Design review of the part built by this model. Coordinates are the model's own, in mm. A direction names the side the tool comes from. Coordinates: 2 decimals unless noted, no trailing zeros. Order: outer loops, then holes, each group sorted by start corner. A loop starts at its lowest first (then second) coordinate and runs counter-clockwise, first axis right, second up. Notation, with made-up numbers: M 59,45.5 L 93,45.5 A18 ccw 93,69.5 Z; hole C 81.5,-30.75 d11. An arc over 180 degrees is marked long. Answer as a JSON object with one key per item and string values.
from build123d import *

# Parameters (mm, degrees)
SKETCH1_W               = 40.3
SKETCH1_H               = 19.5
BOSS_EXTRUDE1_DEPTH     = 27
SKETCH2_W               = 54
SKETCH2_H               = 19.5
BOSS_EXTRUDE2_DEPTH     = 2.5
SKETCH3_W               = 40.3
SKETCH3_H               = 19.5
BOSS_EXTRUDE3_DEPTH     = 6.5
SKETCH4_R               = 2.75
BOSS_EXTRUDE4_DEPTH     = 8
CUT_EXTRUDE1_DEPTH      = 42.162027404
CUT_EXTRUDE1_DEPTH_BACK = 42.162027404
SKETCH5_R               = 2
BOSS_EXTRUDE5_DEPTH     = 3
SKETCH7_R               = 6.5
BOSS_EXTRUDE6_DEPTH     = 2
BOSS_EXTRUDE7_DEPTH     = 3


with BuildPart() as part:
    # Sketch1 → Boss-Extrude1 (new body)
    with BuildSketch(Plane(origin=(0, 0, 0), x_dir=(1, 0, 0), z_dir=(0, 1, 0))):
        Rectangle(SKETCH1_W, SKETCH1_H)
    extrude(amount=BOSS_EXTRUDE1_DEPTH)

    # Sketch2 → Boss-Extrude2 (add)
    with BuildSketch(Plane(origin=(0, 27, 0), x_dir=(1, 0, 0), z_dir=(0, 1, 0))):
        Rectangle(SKETCH2_W, SKETCH2_H)
    extrude(amount=BOSS_EXTRUDE2_DEPTH)

    # Sketch3 → Boss-Extrude3 (add)
    with BuildSketch(Plane(origin=(0, 29.5, 0), x_dir=(1, 0, 0), z_dir=(0, 1, 0))):
        Rectangle(SKETCH3_W, SKETCH3_H)
    extrude(amount=BOSS_EXTRUDE3_DEPTH)

    # Sketch4 → Boss-Extrude4 (add)
    with BuildSketch(Plane(origin=(0, 36, 0), x_dir=(1, 0, 0), z_dir=(0, 1, 0))):
        with Locations(Location((9.85, 0, 0), (0, 0, 270))):
            Circle(SKETCH4_R)
    extrude(amount=BOSS_EXTRUDE4_DEPTH)

    # Sketch5 → Cut-Extrude1 (cut, two sides: drawn at the far end of the back side and taken through both)
    with BuildSketch(Plane(origin=(0, 29.5, 0), x_dir=(1, 0, 0), z_dir=(0, 1, 0)).offset(-CUT_EXTRUDE1_DEPTH_BACK)):
        with Locations(Location((-24.315, 5, 0), (0, 0, 270))):
            Circle(SKETCH5_R)
        with Locations(Location((-24.315, -5, 0), (0, 0, 270))):
            Circle(SKETCH5_R)
        with Locations(Location((24.315, -5, 0), (0, 0, 270))):
            Circle(SKETCH5_R)
        with Locations(Location((24.315, 5, 0), (0, 0, 270))):
            Circle(SKETCH5_R)
    extrude(amount=CUT_EXTRUDE1_DEPTH + CUT_EXTRUDE1_DEPTH_BACK, mode=Mode.SUBTRACT)

    # Sketch6 → Boss-Extrude5 (add)
    with BuildSketch(Plane(origin=(0, 36, 0), x_dir=(1, 0, 0), z_dir=(0, 1, 0))):
        with BuildLine():
            Line((9.85, -9.75), (-13.85, -9.75))
            Line((-13.85, -9.75), (-13.85, 9.75))
            Line((-13.85, 9.75), (9.85, 9.75))
            ThreePointArc((9.85, 9.75), (19.6, 0), (9.85, -9.75))
        make_face()
    extrude(amount=BOSS_EXTRUDE5_DEPTH)

    # Sketch7 → Boss-Extrude6 (add)
    with BuildSketch(Plane(origin=(0, 39, 0), x_dir=(1, 0, 0), z_dir=(0, 1, 0))):
        with Locations(Location((9.85, 0, 0), (0, 0, 270))):
            Circle(SKETCH7_R)
    extrude(amount=BOSS_EXTRUDE6_DEPTH)

    # Sketch8 → Boss-Extrude7 (add)
    with BuildSketch(Plane(origin=(0, 36, 0), x_dir=(1, 0, 0), z_dir=(0, 1, 0))):
        with BuildLine():
            Line((-13.85, 4.510933332), (-13.85, -4.510933332))
            ThreePointArc((-13.85, -4.510933332), (-15.530301972, 0), (-13.85, 4.510933332))
        make_face()
    extrude(amount=BOSS_EXTRUDE7_DEPTH)


solid = part.part
1) Tool access review of faces 4 (the flat face through (24, 29.5, 0)), 5 (the cylindrical face through (19.598, 37.479, -0.214)), 6 (the cylindrical face through (-15.53, 37.48, 0.07)): name each direction out of +Z, -Z, +X, -X, +Y, -Y from which nothing blocks a thin tool from reaching the whole face with its end or side.
Taken from the geometry:
{"face 4": "+Z, -Z, +X, +Y", "face 5": "+X, +Y", "face 6": "-X, +Y"}
2) Add section C-C (x = 6). State the section outline as (y, z) points, and give its area (3 significant figures).
Taken from the geometry:
{"outline": "M 0,-9.75 L 39,-9.75 L 39,-5.24 L 41,-5.24 L 41,5.24 L 39,5.24 L 39,9.75 L 0,9.75 Z", "area": "781 mm2"}
3) Mouldability with a two-part tool opening along Z and no side actions: class faces 1 (the cylindrical face through (-22.33, 28.23, -5.26)), 2 (the flat face through (20.15, 13, 0)), 3 (the flat face through (0, 19, -9.75)) as released by +Z, released by -Z, zero draft, split by the parting line, or undercut.
Taken from the geometry:
{"face 1": "undercut", "face 2": "zero draft", "face 3": "released by -Z"}
4) Add section A-A (z = 0). State the section outline as (x, y) points.
Taken from the geometry:
{"outline": "M -27,27 L -20.15,27 L -20.15,0 L 20.15,0 L 20.15,27 L 27,27 L 27,29.5 L 20.15,29.5 L 20.15,36 L 19.6,36 L 19.6,39 L 16.35,39 L 16.35,41 L 12.6,41 L 12.6,44 L 7.1,44 L 7.1,41 L 3.35,41 L 3.35,39 L -15.53,39 L -15.53,36 L -20.15,36 L -20.15,29.5 L -27,29.5 Z"}
5) Insertion check: pin 1 Ø8 at (x, z) = (-5, -3.5) entering from -Y; pin 2 Ø2 at (x, z) = (-23, -0.5) entering from -Y; pin 3 Ø10 at (x, z) = (-21, 6.5) entering from +Y; pin 4 Ø6 at (y, z) = (7, 5) entering from +X. Each pin has a flat end and moves straight along its axis. Give the tip position at first contact, or say it passes through.
Taken from the geometry:
{"pin 1": "stops at y = 0", "pin 2": "stops at y = 27", "pin 3": "stops at y = 36", "pin 4": "stops at x = 20.15"}
6) Add section B-B (z = 5.25). State the section outline as (x, y) points, and give its area (3 significant figures).
Taken from the geometry:
{"outline": "M -27,27 L -26.3,27 L -26.3,29.5 L -27,29.5 Z; M -22.33,27 L -20.15,27 L -20.15,0 L 20.15,0 L 20.15,27 L 22.33,27 L 22.33,29.5 L 20.15,29.5 L 20.15,36 L 18.07,36 L 18.07,39 L 13.68,39 L 13.68,41 L 6.02,41 L 6.02,39 L -13.85,39 L -13.85,36 L -20.15,36 L -20.15,29.5 L -22.33,29.5 Z; M 26.3,27 L 27,27 L 27,29.5 L 26.3,29.5 Z", "area": "1,580 mm2"}
7) Add section D-D (y = 25). State the section outline as (x, z) points.
Taken from the geometry:
{"outline": "M -20.15,-9.75 L 20.15,-9.75 L 20.15,9.75 L -20.15,9.75 Z"}
8) To check wall thickness, follow L1, parallel to X at y = 28.05, z = 5 (3 decimals); L2, parallel to X at y = 35, z = 4; L3, parallel to Y at x = -1, z = -6.5. State the ranges of each line that lie inside material, in increasing order.
Taken from the geometry:
{"L1": "x = -27 to -26.315, -22.315 to 22.315, 26.315 to 27", "L2": "x = -20.15 to 20.15", "L3": "y = 0 to 39"}
